Source: CAD feature listing. Evaluate the final solid. Frame: model axes, mm. A direction names the side the tool comes from. Coordinates: 2 decimals unless noted, no trailing zeros. Write each loop counter-clockwise with the first axis right and the second up, starting at its lowest first coordinate (ties: lowest second). Pieces come first, ordered by that corner, then holes. Notation, with made-up numbers: (22, 78) -> (57, 78) arc R26 cw to (57, 106) -> close; hole circle Ø9 at (-2, 63.5). An arc over 180 degrees is marked (long way). Write item = value, one per line.
Autodesk Fusion 360 part; units mm, degrees
sketch "Sketch1" plane through (0, 0, 0) normal (0, 1, 0) x (1, 0, 0)
  line L0 (20, -20) -> (-20, -20)
  line L1 (-20, -20) -> (-20, 20)
  line L2 (-20, 20) -> (20, 20)
  line L3 (20, 20) -> (20, -20)
  line L4 (20, -20) -> (-20, 20) construction
  line L5 (-20, -20) -> (20, 20) construction
  line L6 (-20, 4) -> (-15, 4)
  line L7 (-15, 4) -> (-15, -4)
  line L8 (-15, -4) -> (-20, -4)
  line L9 (-20, -4) -> (-20, 4)
  line L10 (-4, 20) -> (4, 20)
  line L11 (4, 20) -> (4, 15)
  line L12 (4, 15) -> (-4, 15)
  line L13 (-4, 15) -> (-4, 20)
  line L14 (20, 4) -> (15, 4)
  line L15 (15, 4) -> (15, -4)
  line L16 (15, -4) -> (20, -4)
  line L17 (20, -4) -> (20, 4)
  line L18 (-4, -20) -> (4, -20)
  line L19 (4, -20) -> (4, -15)
  line L20 (4, -15) -> (-4, -15)
  line L21 (-4, -15) -> (-4, -20)
  dimension "d1" = 40
  dimension "d2" = 40
  dimension "d3" = 5
  dimension "d4" = 8
  dimension "d5" = 16
  dimension "d6" = 5
  dimension "d7" = 16
  dimension "d8" = 8
  dimension "d9" = 5
  dimension "d10" = 5
  dimension "d11" = 8
  dimension "d12" = 8
  dimension "d13" = 16
  dimension "d14" = 16
extrude "Extrude1" add sketch "Sketch1" against normal blind 3 contours L0 L1 L2 L3 L6 L7 L8 L11 L12 L13 L14 L15 L16 L19 L20 L21
extrude "Extrude2" add sketch "Sketch1" against normal blind 8 contours L0 L18 L19 L20 L21 | L3 L14 L15 L16 L17 | L1 L6 L7 L8 L9 | L2 L10 L11 L12 L13
hole "Hole1" at (0, 0, 0) direction (0, -1, 0) diameter 9 depth 30 tip angle 118
fillet "Fillet1" radius 4 4 edges at (20, -1.5, -20) (-20, -1.5, -20) (20, -1.5, 20) (-20, -1.5, 20)
sketch "Sketch2" plane through (0, 0, 0) normal (0, 0, 1) x (1, 0, 0)
sketch "Sketch3" plane through (0, 0, 0) normal (0, 1, 0) x (1, 0, 0)
  line L0 (-10.5, 20) -> (10.5, 20)
  line L1 (10.5, 20) -> (10.5, 8)
  line L2 (10.5, 8) -> (-10.5, 8)
  line L3 (-10.5, 8) -> (-10.5, 20)
  line L4 (-20, -20) -> (-20, 20)
  dimension "d26" = 21
  dimension "d27" = 9.5
  dimension "d28" = 12
extrude "Extrude3" add sketch "Sketch3" along normal blind 80
sketch "Sketch4" plane through (0, 0, -8) normal (0, 0, 1) x (1, 0, 0)
  line L0 (-10.5, 0) -> (10.5, 0)
  line L1 (10.5, 0) -> (10.5, 80)
  line L2 (10.5, 80) -> (-10.5, 80)
  line L3 (-10.5, 80) -> (-10.5, 0)
  line L4 (-10.5, 80) -> (10.5, 80)
  line L5 (10.5, 80) -> (10.5, 59)
  line L6 (10.5, 59) -> (-10.5, 59)
  line L7 (-10.5, 59) -> (-10.5, 80)
  line L8 (8.5, 78) -> (8.5, 61)
  line L9 (8.5, 61) -> (-8.5, 61)
  line L10 (-8.5, 61) -> (-8.5, 78)
  line L11 (-8.5, 78) -> (8.5, 78)
  line L12 (-8.5, 78) -> (8.5, 78)
  line L13 (8.5, 78) -> (8.5, 64.8708)
  line L14 (-8.5, 64.8708) -> (-8.5, 78)
  line L15 (-8.5, 61) -> (8.5, 61)
  line L16 (8.5, 61) -> (8.5, 70.3993)
  line L17 (8.5, 70.3993) -> (-8.5, 70.3993)
  line L18 (-8.5, 70.3993) -> (-8.5, 61)
  point P0 (-7.5, 64)
  point P1 (7.5, 64)
  dimension "d29" = 21
  dimension "d30" = 21
  dimension "d31" = 2
  dimension "d34" = 5
  dimension "d35" = 15
  dimension "d36" = 3
extrude "Extrude6" add sketch "Sketch4" along normal blind 50 contours L1 L2 L3 L4 L5 L6 L7 | L8 L10 L11 L12 L13 L14 L17 | L8 L9 L10 L13 L14 L15 L16 L17 L18
sketch "Sketch7" plane through (0, 0, 42) normal (0, 0, 1) x (1, 0, 0)
  line L0 (-10.5, 59) -> (10.5, 59)
  line L1 (10.5, 59) -> (10.5, 80)
  line L2 (10.5, 80) -> (-10.5, 80)
  line L3 (-10.5, 80) -> (-10.5, 59)
  line L4 (-10.5, 80) -> (10.5, 80)
  line L5 (10.5, 80) -> (10.5, 59)
  line L6 (10.5, 59) -> (-10.5, 59)
  line L7 (-10.5, 59) -> (-10.5, 80)
  line L8 (8.5, 61) -> (-8.5, 61)
  line L9 (-8.5, 61) -> (-8.5, 78)
  line L10 (-8.5, 78) -> (8.5, 78)
  line L11 (8.5, 78) -> (8.5, 61)
  line L12 (-8.5, 78) -> (2.604, 78)
  line L13 (2.604, 78) -> (2.604, 61)
  line L14 (2.604, 61) -> (-8.5, 61)
  line L15 (-8.5, 61) -> (-8.5, 78)
  point P0 (5.5, 77)
  point P1 (5.5, 62)
  point P2 (-33, 92)
  dimension "d55" = 2
  dimension "d58" = 5
  dimension "d59" = 15
  dimension "d60" = 3
extrude "Extrude7" cut sketch "Sketch7" against normal blind 3 contours L8 L9 L10 L12 L13 L14 L15
sketch "Sketch8" plane through (0, 0, -20) normal (0, 0, -1) x (-1, 0, 0)
  line L0 (16, -3) -> (16, 0)
  line L1 (16, 0) -> (10.5, 0)
  line L2 (10.5, 0) -> (10.5, 80)
  line L3 (10.5, 80) -> (-10.5, 80)
  line L4 (-10.5, 80) -> (-10.5, 0)
  line L5 (-10.5, 0) -> (-16, 0)
  line L6 (-16, 0) -> (-16, -3)
  line L7 (-16, -3) -> (-4, -3)
  line L8 (-4, -3) -> (-4, -8)
  line L9 (-4, -8) -> (4, -8)
  line L10 (4, -8) -> (4, -3)
  line L11 (4, -3) -> (16, -3)
  point P0 (-5.5, 77)
  point P1 (-5.5, 62)
  dimension "d61" = 3
  dimension "d62" = 15
  dimension "d63" = 5
hole "Hole5" at (5.5, 62, -20) at (5.5, 77, -20) direction (0, 0, 1) diameter 3 depth 75 tip angle 118 counterbore diameter 5 counterbore depth 59
sketch "Sketch9" plane through (0, -3, 0) normal (0, -1, 0) x (1, 0, 0)
  arc A0 (-16, 20) -> (-20, 16) centre (-16, 16) ccw
  line L0 (-20, 16) -> (-20, 4)
  line L1 (-20, 4) -> (-15, 4)
  line L2 (-15, 4) -> (-15, -4)
  line L3 (-15, -4) -> (-20, -4)
  line L4 (-20, -4) -> (-20, -16)
  arc A1 (-20, -16) -> (-16, -20) centre (-16, -16) ccw
  line L5 (-16, -20) -> (-4, -20)
  line L6 (-4, -20) -> (-4, -15)
  line L7 (-4, -15) -> (4, -15)
  line L8 (4, -15) -> (4, -20)
  line L9 (4, -20) -> (16, -20)
  arc A2 (16, -20) -> (20, -16) centre (16, -16) ccw
  line L10 (20, -16) -> (20, -4)
  line L11 (20, -4) -> (15, -4)
  line L12 (15, -4) -> (15, 4)
  line L13 (15, 4) -> (20, 4)
  line L14 (20, 4) -> (20, 16)
  arc A3 (20, 16) -> (16, 20) centre (16, 16) ccw
  line L15 (16, 20) -> (4, 20)
  line L16 (4, 20) -> (4, 15)
  line L17 (4, 15) -> (-4, 15)
  line L18 (-4, 15) -> (-4, 20)
  line L19 (-4, 20) -> (-16, 20)
  circle A4 centre (0, 0) radius 4.5
  point P0 (2, 0)
sketch "Sketch10" plane through (0, -3, 0) normal (0, -1, 0) x (1, 0, 0)
  circle A0 centre (0, 0) radius 4.5
hole "Hole6" at (0, -3, 0) direction (0, 1, 0) diameter 10 depth 90 tip angle 118
equation "d6 = d3"
equation "d7 = d5"
equation "d8 = d4"
equation "d9 = d3"
equation "d10 = d3"
equation "d11 = d4"
equation "d12 = d4"
equation "d13 = d7"
equation "d14 = d7"
1) Cut plane B-B, the plane x = 0. Output: boundary loops of the cut face in (y, z), and give its area (3 significant figures).
Answer block:
outline = (-8, -20) -> (80, -20) -> (80, -5) -> (59, -5) -> (59, -8) -> (0, -8) -> (0, -5) -> (-3, -5) -> (-3, -15) -> (-8, -15) -> close; (-8, 15) -> (-3, 15) -> (-3, 5) -> (0, 5) -> (0, 20) -> (-8, 20) -> close; (59, 5) -> (80, 5) -> (80, 42) -> (78, 42) -> (78, 39) -> (61, 39) -> (61, 42) -> (59, 42) -> close
area = 1,890 mm2
2) Cut plane A-A, the plane z = 6.5. Output: boundary loops of the cut face in (x, y), and give its area (3 significant figures).
Answer block:
outline = (-20, -3) -> (20, -3) -> (20, 0) -> (-20, 0) -> close; (-10.5, 59) -> (10.5, 59) -> (10.5, 80) -> (-10.5, 80) -> close; hole circle Ø5 at (5.5, 62); hole circle Ø5 at (5.5, 77)
area = 522 mm2
3) Material intervals for probe 1 along Y at (x, z) = (5.5, 3); probe 2 along X at (y, z) = (62, 40.6); probe 3 along Y at (x, z) = (-6, -3), sorted ascending. Write a range as [from, to].
Answer block:
probe_1 = [-3, 0], [59, 59.5], [64.5, 74.5], [79.5, 80]
probe_2 = [-10.5, -8.5], [2.6, 4], [7, 10.5]
probe_3 = [-3, 0], [59, 80]
4) Cut plane C-C, the plane y = 77. Output: boundary loops of the cut face in (x, z), and give its area (3 significant figures).
Answer block:
outline = (-10.5, -20) -> (3, -20) -> (3, -4) arc R5 cw (long way) to (3, 4) -> (3, 39) -> (4, 39) -> (4, 42) -> (2.6, 42) -> (2.6, 39) -> (-8.5, 39) -> (-8.5, 42) -> (-10.5, 42) -> close; (7, 39) -> (8, 39) -> (8, -20) -> (10.5, -20) -> (10.5, 42) -> (7, 42) -> close
area = 897 mm2
5) Cut plane D-D, the plane z = 31. Output: boundary loops of the cut face in (x, y).
Answer block:
outline = (-10.5, 59) -> (10.5, 59) -> (10.5, 80) -> (-10.5, 80) -> close; hole circle Ø5 at (5.5, 62); hole circle Ø5 at (5.5, 77)
6) Reachability of faces 1 (the flat face through (0, -5, -15)), 2 (the flat face through (-4, -5, -17)), 3 (the flat face through (-17, -5, 4)), 4 (the flat face through (15, -5, 0)), 5 (the flat face through (2.604, 70, 41)) from +Z, -Z, +X, -X, +Y, -Y: full face, straight path, thin tool, end or side. Return the list, or none.
Answer block:
face_1 = +X, -X, -Y
face_2 = +Z, -Z, -X, -Y
face_3 = +Z, +X, -X, -Y
face_4 = +Z, -Z, -Y
face_5 = +Z
7) Pull-direction query (X, two-part tool) for faces 6 (the flat face through (17, -5, 4)), 7 (the cylindrical face through (7.94, 61.46, 9.91)), 8 (the flat face through (7, 78, 39)), 9 (the cylindrical face through (18.797, -1.521, -18.859)); classes: +X half, -X half, draft (parallel to the pull), parting line (faces both ways), or undercut.
Answer block:
face_6 = draft
face_7 = undercut
face_8 = undercut
face_9 = +X half
8) First-contact query: pin 1 Ø1.5 at (x, y) = (6.5, 77.5) entering from -Z; pin 2 Ø12 at (x, z) = (4.5, 8) entering from -Y; pin 3 Ø5.5 at (x, y) = (0.5, -5) entering from +Z; pin 4 Ø6 at (x, z) = (0, 0) entering from -Y. Flat tips, straight axial feed; report the tip coordinate or a pass-through.
Answer block:
pin_1 = 39
pin_2 = -3
pin_3 = 20
pin_4 = through
